Read the model definition and answer for the solid it produces. Units are mm, in the model's axes. Coordinates: 2 decimals unless noted, no trailing zeros. Order: outer loops, then holes, each group sorted by start corner. A loop starts at its lowest first (then second) coordinate and runs counter-clockwise, first axis right, second up. Notation, with made-up numbers: M 60.5,20 L 84.5,20 A24 ccw 84.5,46 Z; hole C 0,27.5 d9. An arc over 180 degrees is marked long. Use a Markdown table: item, result. Add a question column.
1) Find section A-A on x = -235. Write down the section's boundary in (y, z).
2) Find section C-C on x = -85. Write down the section's boundary in (y, z).
3) Find section B-B on y = 1.7. Count the separate pieces of the cut face and the enclosed holes in it, plus the area to 3 significant figures.
4) Find the intervals of material crossed by probe 1 along Z at (x, y) = (-235, 3.3); probe 2 along X at (y, z) = (0.75, -25); probe 3 along Z at (x, y) = (-15, 3.9), in increasing order. Write a range as [from, to].
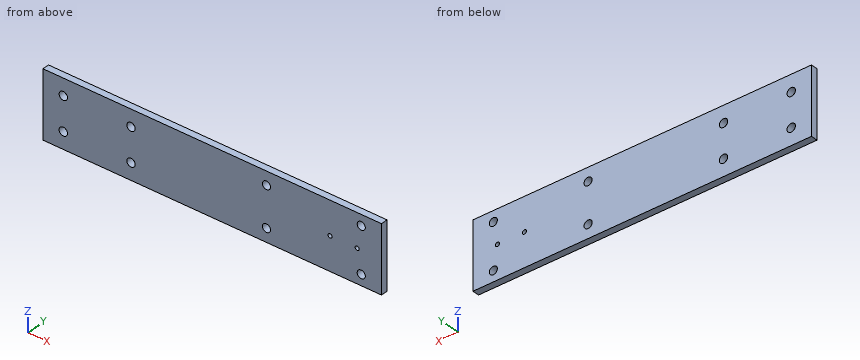
Autodesk Inventor part; units mm, degrees
ref_plane "YZ-Ebene" through (0, 0, 0) normal (1, 0, 0) x (0, 1, 0)
ref_plane "XZ-Ebene" through (0, 0, 0) normal (0, 1, 0) x (-1, 0, 0)
ref_plane "XY-Ebene" through (0, 0, 0) normal (0, 0, 1) x (1, 0, 0)
sketch "Skizze1" plane through (0, 0, 0) normal (0, 1, 0) x (-1, 0, 0)
  line L0 (250, -50) -> (0, -50)
  line L1 (0, -50) -> (0, 0)
  line L2 (0, 0) -> (250, 0)
  line L3 (250, 0) -> (250, -50)
  dimension "d0" = 250
  dimension "d1" = 50
extrude "Extrusion1" add sketch "Skizze1" along normal blind 5
sketch "Skizze2" plane through (0, 5, 0) normal (0, 1, 0) x (1, 0, 0)
  circle A0 centre (-235, 37.5) radius 3.1
  circle A1 centre (-185, 37.5) radius 3.1
  circle A2 centre (-235, 12.5) radius 3.1
  circle A3 centre (-185, 12.5) radius 3.1
  line L0 (0, 50) -> (-250, 50)
  line L1 (-250, 50) -> (-250, 0)
  point P0 (0, 0)
  dimension "d4" = 6.2
  dimension "d5" = 6.2
  dimension "d6" = 6.2
  dimension "d7" = 6.2
  dimension "d8" = 12.5
  dimension "d9" = 25
  dimension "d10" = 25
  dimension "d11" = 50
  dimension "d12" = 50
  dimension "d13" = 15
  dimension "d14" = 15
  dimension "d15" = 12.5
extrude "Extrusion2" cut sketch "Skizze2" against normal blind 6
sketch "Skizze3" plane through (0, 5, 0) normal (0, 1, 0) x (1, 0, 0)
  circle A0 centre (-15, 42) radius 3
  circle A1 centre (-15, 8) radius 3
  circle A2 centre (-84.9714, 10) radius 3
  circle A3 centre (-85, 40) radius 3
  line L0 (0, 0) -> (0, 50)
  line L1 (0, 50) -> (-250, 50)
  dimension "d18" = 6
  dimension "d19" = 6
  dimension "d20" = 6
  dimension "d21" = 6
  dimension "d22" = 15
  dimension "d23" = 15
  dimension "d24" = 70
  dimension "d25" = 70
  dimension "d26" = 34
  dimension "d27" = 30
  dimension "d28" = 10
  dimension "d29" = 8
extrude "Extrusion3" cut sketch "Skizze3" against normal blind 10
sketch "Skizze4" plane through (0, 5, 0) normal (0, 1, 0) x (1, 0, 0)
  circle A0 centre (-38, 25) radius 1.5
  circle A1 centre (-18, 25) radius 1.5
  line L0 (0, 50) -> (-250, 50)
  line L1 (0, 0) -> (0, 50)
  dimension "d32" = 3
  dimension "d33" = 3
  dimension "d34" = 25
  dimension "d35" = 25
  dimension "d36" = 18
  dimension "d37" = 20
extrude "Extrusion4" cut sketch "Skizze4" against normal blind 10
properties part number "adapter_chipshouter"
Check result:
| question | item | result |
|---|---|---|
| 1 | outline | M 0,-50 L 5,-50 L 5,-40.6 L 0,-40.6 Z; M 0,-34.4 L 5,-34.4 L 5,-15.6 L 0,-15.6 Z; M 0,-9.4 L 5,-9.4 L 5,0 L 0,0 Z |
| 2 | outline | M 0,-50 L 5,-50 L 5,-43 L 0,-43 Z; M 0,-37 L 5,-37 L 5,-13 L 0,-13 Z; M 0,-7 L 5,-7 L 5,0 L 0,0 Z |
| 3 | separate pieces | 1 |
| 3 | enclosed holes | 10 |
| 3 | area | 12,300 mm2 |
| 4 | probe 1 | z = [-50, -40.6], [-34.4, -15.6], [-9.4, 0] |
| 4 | probe 2 | x = [-250, -39.5], [-36.5, -19.5], [-16.5, 0] |
| 4 | probe 3 | z = [-50, -45], [-39, -11], [-5, 0] |
